Answer from the drawing. Dimensions are ordinates in mm from the lowest x, y and z of the part. A direction names the side the tool comes from. Give positions to 0.01 mm unless a question says otherwise; leave off trailing zeros. Order: outer loops, then holes, each group sorted by start corner. A loop starts at its lowest first (then second) coordinate and runs counter-clockwise, first axis right, second up. Notation, with made-up numbers: (59.5, 19) - (107.5, 19) arc R6 cw to (107.5, 29) - close; hole circle Ø7 at (84, 27.5). An arc over 180 degrees is marked (long way). Answer in a Markdown table with one row per item.
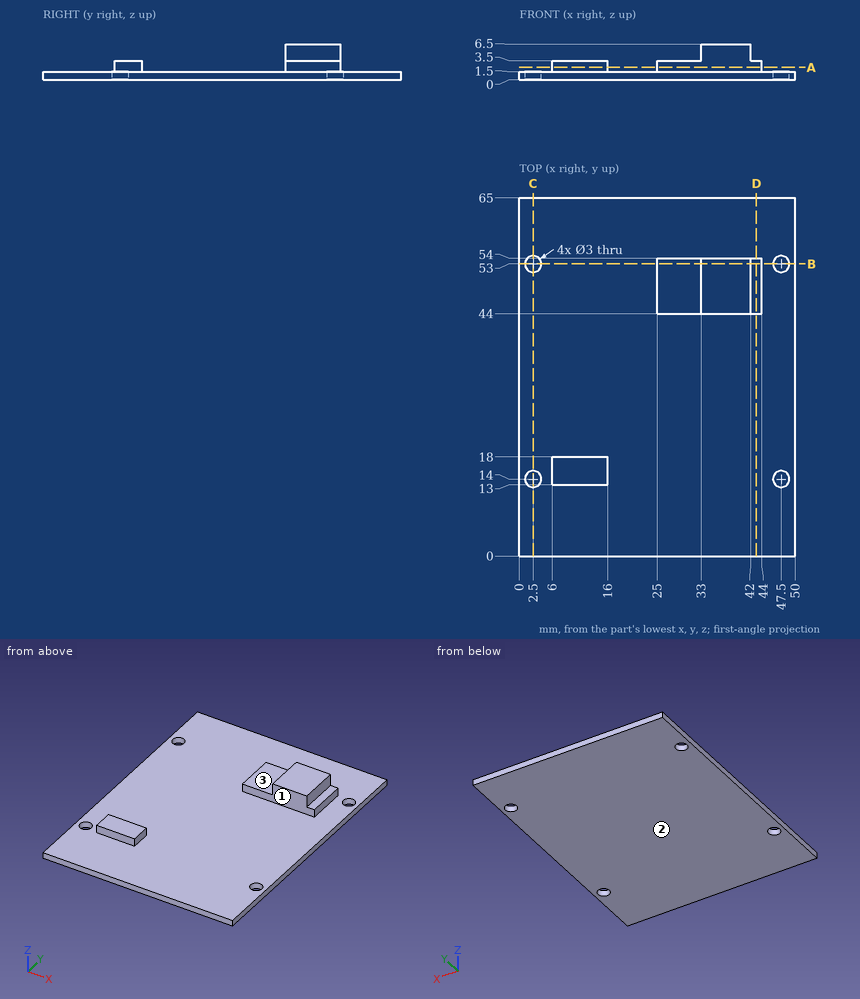
Item 1: Find section C-C on x = 2.5. Write down the section's boundary in (y, z).
Answer block:
| item | result |
|---|---|
| outline | (0, 0) - (12.5, 0) - (12.5, 1.5) - (0, 1.5) - close; (15.5, 0) - (51.5, 0) - (51.5, 1.5) - (15.5, 1.5) - close; (54.5, 0) - (65, 0) - (65, 1.5) - (54.5, 1.5) - close |
Item 2: Which of the six approach directions +Z, -Z, +X, -X, +Y, -Y give full straight-line access (tool end or side, diameter ignored) to the marked faces 1, 2 and 3?
Answer block:
| item | result |
|---|---|
| face 1 | +Z, +X, -X, -Y |
| face 2 | -Z, +X, -X, +Y, -Y |
| face 3 | +Z, -X, +Y, -Y |
Item 3: Find section B-B on y = 53. Write down the section's boundary in (x, z), then the cut area to 3 significant figures.
Answer block:
| item | result |
|---|---|
| outline | (0, 0) - (1, 0) - (1, 1.5) - (0, 1.5) - close; (4, 0) - (46, 0) - (46, 1.5) - (44, 1.5) - (44, 3.5) - (42, 3.5) - (42, 6.5) - (33, 6.5) - (33, 3.5) - (25, 3.5) - (25, 1.5) - (4, 1.5) - close; (49, 0) - (50, 0) - (50, 1.5) - (49, 1.5) - close |
| area | 131 mm² |
Item 4: Consider line 1 (Y direction, x = 2.5, z = 1); line 2 (X direction, y = 53, z = 1.15); line 3 (Z direction, x = 36.5, y = 6). Determine where each line is inside the solid, lowest interval first.
Answer block:
| item | result |
|---|---|
| line 1 | 0 to 12.5, 15.5 to 51.5, 54.5 to 65 |
| line 2 | 0 to 1, 4 to 46, 49 to 50 |
| line 3 | 0 to 1.5 |
Item 5: Find section D-D on x = 43. Write down the section's boundary in (y, z).
Answer block:
| item | result |
|---|---|
| outline | (0, 0) - (65, 0) - (65, 1.5) - (54, 1.5) - (54, 3.5) - (44, 3.5) - (44, 1.5) - (0, 1.5) - close |
Item 6: Find section A-A on z = 2.25. Write down the section's boundary in (x, y), then the cut area to 3 significant figures.
Answer block:
| item | result |
|---|---|
| outline | (6, 13) - (16, 13) - (16, 18) - (6, 18) - close; (25, 44) - (44, 44) - (44, 54) - (25, 54) - close |
| area | 240 mm² |
Item 7: Each of these flat-tipped pins is pushed along its axis until it touches: P1, Ø1.5, axis at x = 10, y = 16, coming from the +Z side; P2, Ø0.6, axis at y = 50, z = 2.5, coming from the -X side; P3, Ø1.6, axis at y = 14.5, z = 3, coming from the +X side. Where does it stop, or does it pass through?
Answer block:
| item | result |
|---|---|
| P1 | z = 3.5 |
| P2 | x = 25 |
| P3 | x = 16 |
